Autodesk Inventor part; units mm, degrees
ref_plane "YZ Plane" through (0, 0, 0) normal (1, 0, 0) x (0, 1, 0)
ref_plane "XZ Plane" through (0, 0, 0) normal (0, 1, 0) x (-1, 0, 0)
ref_plane "XY Plane" through (0, 0, 0) normal (0, 0, 1) x (1, 0, 0)
sketch "Sketch1" plane through (0, 0, 0) normal (0, 0, 1) x (1, 0, 0)
  line L0 (-170, 0) -> (-170, 12.5)
  line L1 (-170, 12.5) -> (-160, 12.5)
  line L2 (-160, 12.5) -> (-160, 15.5)
  line L3 (-160, 15.5) -> (-50, 15.5)
  line L4 (-50, 15.5) -> (-50, 12.5)
  line L5 (-50, 12.5) -> (0, 12.5)
  line L6 (-238, 0) -> (238, 0)
  line L7 (-170, 0) -> (-170, -12.5)
  line L8 (-170, -12.5) -> (-160, -12.5)
  line L9 (-160, -12.5) -> (-160, -15.5)
  line L10 (-160, -15.5) -> (-50, -15.5)
  line L11 (-50, -15.5) -> (-50, -12.5)
  line L12 (-50, -12.5) -> (0, -12.5)
  line L13 (0, -21.7) -> (0, 21.7)
  line L14 (170, 0) -> (170, 12.5)
  line L15 (170, 12.5) -> (160, 12.5)
  line L16 (160, 12.5) -> (160, 15.5)
  line L17 (160, 15.5) -> (50, 15.5)
  line L18 (50, 15.5) -> (50, 12.5)
  line L19 (50, 12.5) -> (0, 12.5)
  line L20 (170, 0) -> (170, -12.5)
  line L21 (170, -12.5) -> (160, -12.5)
  line L22 (160, -12.5) -> (160, -15.5)
  line L23 (160, -15.5) -> (50, -15.5)
  line L24 (50, -15.5) -> (50, -12.5)
  line L25 (50, -12.5) -> (0, -12.5)
  point P0 (0, 0)
  point P1 (50, 14)
  point P2 (-50, 14)
  point P3 (-165, -12.5)
  point P4 (-165, 12.5)
  dimension "d0" = 3
  dimension "d2" = 100
  dimension "d3" = 10
  dimension "d4" = 110
  dimension "d5" = 25
extrude "Extrusion1" add sketch "Sketch1" along normal blind 3
fillet "Fillet1" radius 1 8 edges at (-160, 15.5, 1.5) (-50, 15.5, 1.5) (50, 15.5, 1.5) (160, 15.5, 1.5) (160, -15.5, 1.5) (50, -15.5, 1.5) (-50, -15.5, 1.5) (-160, -15.5, 1.5)
properties part number "ConectorPared"
The model under review builds one solid part; all positions refer to its coordinate system, in mm. Coordinates: 2 decimals unless noted, no trailing zeros. Loops run counter-clockwise (first coordinate to the right, second up) from the corner with the lowest first, then second, coordinate; pieces in that order, holes last. Notation, with made-up numbers: (19.5, 74.5) -> (51.5, 74.5) arc R16 ccw to (51.5, 105.5) -> close; hole circle Ø1 at (31, -15.5). An arc over 180 degrees is marked (long way). Answer as CSV lines item,"result".
Item 1: Take a section at B-B, the plane x = -36.5. State the section outline as (y, z) points.
Results below:
outline,"(-12.5, 0) -> (12.5, 0) -> (12.5, 3) -> (-12.5, 3) -> close"
Item 2: For L1, parallel to Y at x = -35, z = 0.3, list the stretches that pass through material, from the lowest coordinate up.
Results below:
L1,"y = -12.5 to 12.5"
Item 3: Insertion check: pin 1 (1.6 mm diameter, centred on y = -14, z = 1.5, fed in from -X); pin 2 (1 mm diameter, centred on x = 46.5, z = 1, fed in from -Y); pin 3 (1.5 mm diameter, centred on x = -22, z = 2, fed in from +Y). Each pin has a flat end and moves straight along its axis. Give the tip position at first contact, or say it passes through.
Results below:
pin 1,"stops at x = -160"
pin 2,"stops at y = -12.5"
pin 3,"stops at y = 12.5"
Item 4: Take a section at A-A, the plane z = 2.45. State the section outline as (x, y) points, and give its area (3 significant figures).
Results below:
outline,"(-170, -12.5) -> (-160, -12.5) -> (-160, -14.5) arc R1 ccw to (-159, -15.5) -> (-51, -15.5) arc R1 ccw to (-50, -14.5) -> (-50, -12.5) -> (50, -12.5) -> (50, -14.5) arc R1 ccw to (51, -15.5) -> (159, -15.5) arc R1 ccw to (160, -14.5) -> (160, -12.5) -> (170, -12.5) -> (170, 12.5) -> (160, 12.5) -> (160, 14.5) arc R1 ccw to (159, 15.5) -> (51, 15.5) arc R1 ccw to (50, 14.5) -> (50, 12.5) -> (-50, 12.5) -> (-50, 14.5) arc R1 ccw to (-51, 15.5) -> (-159, 15.5) arc R1 ccw to (-160, 14.5) -> (-160, 12.5) -> (-170, 12.5) -> close"
area,"9,820 mm2"
